```python
from build123d import *

# Parameters (mm, degrees)
SKETCH1_R           = 5
BOSS_EXTRUDE1_DEPTH = 50
CUT_EXTRUDE1_DEPTH  = 101
CHAMFER1_SIZE       = 0.4


with BuildPart() as part:
    # Sketch1 → Boss-Extrude1 (new body, symmetric)
    with BuildSketch(Plane.XY):
        Circle(SKETCH1_R)
    extrude(amount=BOSS_EXTRUDE1_DEPTH, both=True)

    # Sketch3 → Hole1 (revolve, cut)
    with BuildSketch(Plane(origin=(0, 0, 50), x_dir=(0, -1, 0), z_dir=(1, 0, 0))):
        Polygon((0, 0), (0, 13.85), (1.85, 12), (1.85, 0), align=None)
    hole1 = revolve(axis=Axis((0, 0, 54.244199587), (0, 0, -1)), mode=Mode.SUBTRACT)

    # Mirror7: Hole1 across plane
    add(hole1.mirror(Plane.XY), mode=Mode.SUBTRACT)

    # Sketch4 → Cut-Extrude1 (cut, through all)
    with BuildSketch(Plane.XY.offset(50)):
        with BuildLine():
            Line((-2.374868417, -4.4), (2.374868417, -4.4))
            ThreePointArc((2.374868417, -4.4), (0, -5), (-2.374868417, -4.4))
        make_face()
    extrude(amount=-CUT_EXTRUDE1_DEPTH, mode=Mode.SUBTRACT)

    # Chamfer1
    chamfer1_edges = [part.edges().sort_by_distance(p)[0] for p in [
        (0, 5, -50),
        (0, 5, 50),
        (0, -4.4, -50),
        (0, -4.4, 50),
    ]]
    chamfer(chamfer1_edges, length=CHAMFER1_SIZE)


solid = part.part
```
Could you check a few things on this model? Use its own coordinates, in mm. A direction names the side the tool comes from. Round coordinates to 2 decimals unless told otherwise and drop trailing zeros. Loops run counter-clockwise (first coordinate to the right, second up) from the corner with the lowest first, then second, coordinate; pieces in that order, holes last. Notation, with made-up numbers: (14, -15) - (35, -15) arc R23 cw to (35, 17) - close; hole circle Ø3 at (31, 1). An arc over 180 degrees is marked (long way). Answer in a Markdown table with one row per item. Add a question column.
(1) If we section it at B-B (z = -39): Please give me the cut outline in (x, y).
(2) If we mould it in two halves opening along Y, with no side actions, what happens to faces 4 (the face through (-1, -2, -50)), 5 (the face through (0, 5, 1)), 6 (the face through (0.514, 0.114, -36.677)), 7 (the face through (0, -4.4, 1))? For each: pulls with the +Y half, pulls with the -Y half, needs draft (parallel to the pull), parting line crosses it, or undercut.
(3) I'm going to push flat-ended pins straight in: pin 1 (1 mm diameter, centred on y = -2.5, z = -2.5, fed in from +X); pin 2 (3 mm diameter, centred on x = 0, y = 0, fed in from -Z); pin 3 (2 mm diameter, centred on x = 3, z = -13, fed in from +Y). Where does each tip first touch, or does it pass through?
(4) I need wall thicknesses on line 1 along X through (y, z) = (0, -45.75); line 2 along Y through (x, z) = (0, -41.25); line 3 along X through (y, z) = (2, 42.5). Which ranges of each line are inside material? Lowest first, please.
(5) For faces 1 (the face through (-1, -2, 50)), 2 (the face through (1.806, 0.401, -44.084)), 3 (the face through (1.806, 0.401, 44.084)), which set-ups out of +Z, -Z, +X, -X, +Y, -Y let a thin tool reach every point of the face, with its end or its side?
(6) If we section it at A-A (z = -1.5): Please give me the cut outline in (x, y).
Model answer:
| question | item | result |
|---|---|---|
| 1 | outline | (-2.37, -4.4) - (2.37, -4.4) arc R5 ccw (long way) to start; hole circle Ø3.7 at (0, 0) |
| 2 | face 4 | needs draft |
| 2 | face 5 | parting line crosses it |
| 2 | face 6 | undercut |
| 2 | face 7 | pulls with the -Y half |
| 3 | pin 1 | stops at x = 4.58 |
| 3 | pin 2 | stops at z = -37.65 |
| 3 | pin 3 | stops at y = 4.58 |
| 4 | line 1 | x = -5 to -1.85, 1.85 to 5 |
| 4 | line 2 | y = -4.4 to -1.85, 1.85 to 5 |
| 4 | line 3 | x = -4.58 to 4.58 |
| 5 | face 1 | +Z, +X, -X, +Y, -Y |
| 5 | face 2 | -Z |
| 5 | face 3 | +Z |
| 6 | outline | (-2.37, -4.4) - (2.37, -4.4) arc R5 ccw (long way) to start |
